Verification items for the finished model (mm, model axes). Round coordinates to 2 decimals unless told otherwise and drop trailing zeros. Loops run counter-clockwise (first coordinate to the right, second up) from the corner with the lowest first, then second, coordinate; pieces in that order, holes last. Notation, with made-up numbers: (68, -28.5) - (74, -28.5) arc R4 ccw to (74, -23.5) - close; hole circle Ø2 at (57, -1.5). An arc over 180 degrees is marked (long way). Use CSV: the item, a comma, the result in double quotes.
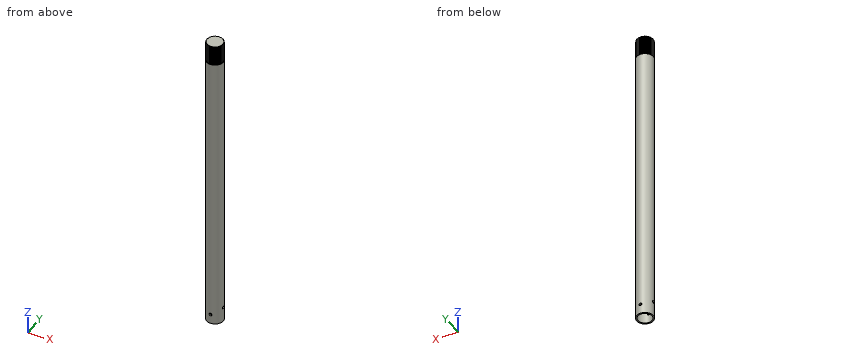
```python
from build123d import *

# Parameters (mm, degrees)
SKETCH5_W               = 1.587499994
SKETCH5_H               = 345.340081988
CUT_EXTRUDE5_DEPTH      = 368.748370511
CUT_EXTRUDE5_DEPTH_BACK = 368.748370511
SKETCH7_R               = 1.5875
CUT_EXTRUDE6_DEPTH      = 368.748370616
CUT_EXTRUDE6_DEPTH_BACK = 368.748370616
SKETCH6_R               = 1.5875
CUT_EXTRUDE7_START      = 367.501582
SKETCH8_R               = 12.7
CUT_EXTRUDE7_DEPTH      = 22.225
SKETCH10_R              = 7.9375
BOSS_EXTRUDE1_DEPTH     = 319.940081988


with BuildPart() as part:
    # Sketch5 → Revolve2 (revolve)
    with BuildSketch(Plane(origin=(0, 0, 0), x_dir=(1, 0, 0), z_dir=(0, 1, 0)), mode=Mode.PRIVATE) as revolve2_sk:
        with Locations((8.731249997, -194.831540994)):
            Rectangle(SKETCH5_W, SKETCH5_H)
    revolve(revolve2_sk.sketch.rotate(Axis((0, 0, 0), (0, 0, 1)), 180), axis=Axis((0, 0, 0), (0, 0, 1)))

    # Sketch7 → Cut-Extrude5 (cut, two sides: drawn at the far end of the back side and taken through both)
    with BuildSketch(Plane(origin=(0, 0, 0), x_dir=(0, 0, -1), z_dir=(1, 0, 0)).offset(-CUT_EXTRUDE5_DEPTH_BACK)):
        with Locations((-39.195999993, 0)):
            Circle(SKETCH7_R)
    extrude(amount=CUT_EXTRUDE5_DEPTH + CUT_EXTRUDE5_DEPTH_BACK, mode=Mode.SUBTRACT)

    # Sketch6 → Cut-Extrude6 (cut, two sides: drawn at the far end of the back side and taken through both)
    with BuildSketch(Plane(origin=(0, 0, 0), x_dir=(1, 0, 0), z_dir=(0, 1, 0)).offset(-CUT_EXTRUDE6_DEPTH_BACK)):
        with Locations(Location((1e-09, -33.163499999, 0), (0, 0, 269.999999955))):
            Circle(SKETCH6_R)
    extrude(amount=CUT_EXTRUDE6_DEPTH + CUT_EXTRUDE6_DEPTH_BACK, mode=Mode.SUBTRACT)

    # Sketch8 → Cut-Extrude7 (cut)
    with BuildSketch(Plane.XY.offset(CUT_EXTRUDE7_START)):
        Circle(SKETCH8_R)
        Polygon((9.235721046, -0.808020891), (8.681700155, -0.254), (8.681700155, 0.254), (9.235721046, 0.808020891), (8.593912259, 1.257420242), (8.505698985, 1.75770258), (8.955098336, 2.399511367), (8.245002688, 2.730634406), (8.071256455, 3.207998257), (8.402379494, 3.918093905), (7.645572882, 4.120879625), (7.391572882, 4.56082053), (7.594358603, 5.317627141), (6.813836213, 5.385914002), (6.487300108, 5.775064579), (6.555586968, 6.555586968), (5.775064579, 6.487300108), (5.385914002, 6.813836213), (5.317627141, 7.594358603), (4.56082053, 7.391572882), (4.120879625, 7.645572882), (3.918093905, 8.402379494), (3.207998257, 8.071256455), (2.730634406, 8.245002688), (2.399511367, 8.955098336), (1.75770258, 8.505698985), (1.257420242, 8.593912259), (0.808020891, 9.235721046), (0.254, 8.681700155), (-0.254, 8.681700155), (-0.808020891, 9.235721046), (-1.257420242, 8.593912259), (-1.75770258, 8.505698985), (-2.399511367, 8.955098336), (-2.730634406, 8.245002688), (-3.207998257, 8.071256455), (-3.918093905, 8.402379494), (-4.120879625, 7.645572882), (-4.56082053, 7.391572882), (-5.317627141, 7.594358603), (-5.385914002, 6.813836213), (-5.775064579, 6.487300108), (-6.555586968, 6.555586968), (-6.487300108, 5.775064579), (-6.813836213, 5.385914002), (-7.594358603, 5.317627141), (-7.391572882, 4.56082053), (-7.645572882, 4.120879625), (-8.402379494, 3.918093905), (-8.071256455, 3.207998257), (-8.245002688, 2.730634406), (-8.955098336, 2.399511367), (-8.505698985, 1.75770258), (-8.593912259, 1.257420242), (-9.235721046, 0.808020891), (-8.681700155, 0.254), (-8.681700155, -0.254), (-9.235721046, -0.808020891), (-8.593912259, -1.257420242), (-8.505698985, -1.75770258), (-8.955098336, -2.399511367), (-8.245002688, -2.730634406), (-8.071256455, -3.207998257), (-8.402379494, -3.918093905), (-7.645572882, -4.120879625), (-7.391572882, -4.56082053), (-7.594358603, -5.317627141), (-6.813836213, -5.385914002), (-6.487300108, -5.775064579), (-6.555586968, -6.555586968), (-5.775064579, -6.487300108), (-5.385914002, -6.813836213), (-5.317627141, -7.594358603), (-4.56082053, -7.391572882), (-4.120879625, -7.645572882), (-3.918093905, -8.402379494), (-3.207998257, -8.071256455), (-2.730634406, -8.245002688), (-2.399511367, -8.955098336), (-1.75770258, -8.505698985), (-1.257420242, -8.593912259), (-0.808020891, -9.235721046), (-0.254, -8.681700155), (0.254, -8.681700155), (0.808020891, -9.235721046), (1.257420242, -8.593912259), (1.75770258, -8.505698985), (2.399511367, -8.955098336), (2.730634406, -8.245002688), (3.207998257, -8.071256455), (3.918093905, -8.402379494), (4.120879625, -7.645572882), (4.56082053, -7.391572882), (5.317627141, -7.594358603), (5.385914002, -6.813836213), (5.775064579, -6.487300108), (6.555586968, -6.555586968), (6.487300108, -5.775064579), (6.813836213, -5.385914002), (7.594358603, -5.317627141), (7.391572882, -4.56082053), (7.645572882, -4.120879625), (8.402379494, -3.918093905), (8.071256455, -3.207998257), (8.245002688, -2.730634406), (8.955098336, -2.399511367), (8.505698985, -1.75770258), (8.593912259, -1.257420242), align=None, mode=Mode.SUBTRACT)
    extrude(amount=-CUT_EXTRUDE7_DEPTH, mode=Mode.SUBTRACT)

    # Sketch10 → Boss-Extrude1 (add)
    with BuildSketch(Plane(origin=(0, 0, 47.5615), x_dir=(-1, 0, 0), z_dir=(0, 0, -1))):
        Circle(SKETCH10_R)
    extrude(amount=-BOSS_EXTRUDE1_DEPTH)


solid = part.part
```
1) Thickness scan on probe 1 along Z at (x, y) = (9.05, 0); probe 2 along Z at (x, y) = (-3.75, 4.25); probe 3 along X at (y, z) = (0.5, 79.5). Record the ranges inside material, lowest first. Write a range as [from, to].
Returned:
probe 1,"z = [22.16, 37.61], [40.78, 345.28]"
probe 2,"z = [47.56, 367.5]"
probe 3,"x = [-9.51, 9.51]"
2) Cross-section at A-A, the plane z = 118. Record the cut outline in (x, y) (3 decimals).
Returned:
outline,"circle Ø19.05 at (0, 0)"
3) Gauge pin test, flat ends, axial feed: pin 1 Ø3 at (y, z) = (6.5, 160) entering from -X; pin 2 Ø5 at (x, z) = (6, 76.5) entering from +Y; pin 3 Ø0.6 at (y, z) = (0, 354) entering from +X; pin 4 Ø3 at (x, z) = (0, 33.16) entering from -Y. Record the tip position at first contact, or that the pin passes through.
Returned:
pin 1,"stops at x = -8.11"
pin 2,"stops at y = 8.86"
pin 3,"stops at x = 8.73"
pin 4,"passes through"
